For this review, take the finished solid that the model builds, in its own axes (mm). Face numbers are marked on the shaded views. A direction names the side the tool comes from. Round coordinates to 2 decimals unless told otherwise and drop trailing zeros. Order: outer loops, then holes, each group sorted by start corner. A loop starts at its lowest first (then second) coordinate and runs counter-clockwise, first axis right, second up. Notation, with made-up numbers: M 44.5,17 L 66.5,17 A31 ccw 66.5,43 Z; hole C 15.25,33.5 d6. An arc over 180 degrees is marked long. Use a Markdown table: item, result.
from build123d import *

# Parameters (mm, degrees)
F3_DEPTH = 25
F2_W     = 14.679278
F2_H     = 9.152961
F4_DEPTH = 25
F5_DEPTH = 25


with BuildPart() as f3:
    # F1 (on Front) → F3 (new body, symmetric)
    with BuildSketch(Plane.XZ):
        with BuildLine():
            Line((15.849059, 25), (-19.900017, 25))
            ThreePointArc((-19.900017, 25), (-23.663126, 21.043852), (-25, 15.75))
            Line((-25, 15.75), (-25, -13.906561))
            Line((-25, -13.906561), (-25, -14.566518))
            ThreePointArc((-25, -14.566518), (-21.671652, -22.024724), (-14.065702, -25))
            Line((-14.065702, -25), (15.273589, -25))
            ThreePointArc((15.273589, -25), (20.913091, -23.706775), (25, -19.611218))
            Line((25, -19.611218), (25, -9.521818))
            Line((25, -9.521818), (25, 15.948113))
            ThreePointArc((25, 15.948113), (22.284826, 22.35471), (15.849059, 25))
        make_face()
        with BuildLine():
            Line((-10.707237, -10.016448), (-10.707237, 0))
            Line((-10.707237, 0), (-10.707237, 10.016448))
            ThreePointArc((-10.707237, 10.016448), (-10.10992, 12.373308), (-8.462171, 14.161184))
            Line((-8.462171, 14.161184), (4.317435, 14.161184))
            Line((4.317435, 14.161184), (5.699014, 14.161184))
            ThreePointArc((5.699014, 14.161184), (8.629785, 12.947219), (9.843749, 10.016448))
            Line((9.843749, 10.016448), (9.843749, 0))
            Line((9.843749, 0), (9.843749, -10.016448))
            ThreePointArc((9.843749, -10.016448), (8.630455, -12.592476), (5.871711, -13.297698))
            Line((5.871711, -13.297698), (-6.907895, -13.297698))
            ThreePointArc((-6.907895, -13.297698), (-9.558442, -12.526508), (-10.707237, -10.016448))
        make_face(mode=Mode.SUBTRACT)
    extrude(amount=F3_DEPTH, both=True)

    # F2 (on Right) → F4 (intersect, symmetric)
    with BuildSketch(Plane.YZ):
        with BuildLine():
            Line((-25, -25), (-7.54655, -25))
            Line((-7.54655, -25), (-7.54655, -10.016448))
            Line((-7.54655, -10.016448), (6.960031, -10.016448))
            Line((6.960031, -10.016448), (6.960031, -25))
            Line((6.960031, -25), (25, -25))
            Line((25, -25), (25, 15.715461))
            ThreePointArc((25, 15.715461), (21.733554, 22.047274), (15.249502, 25))
            Line((15.249502, 25), (-15.145234, 25))
            ThreePointArc((-15.145234, 25), (-21.510489, 22.233155), (-25, 16.233554))
            Line((-25, 16.233554), (-25, -25))
        make_face()
        with Locations((-0.725002, 10.793585)):
            Rectangle(F2_W, F2_H, mode=Mode.SUBTRACT)
    extrude(amount=F4_DEPTH, both=True, mode=Mode.INTERSECT)

    # F0 (on Top) → F5 (intersect, symmetric)
    with BuildSketch(Plane.XY):
        Polygon((25, 25), (-25, 25), (-25, 16.938681), (-13, 16.938681), (-13, -17.136794), (-25, -17.136794), (-25, -25), (25, -25), (25, -16.344341), (13, -16.344341), (13, 16.542453), (25, 16.542453), align=None)
    extrude(amount=F5_DEPTH, both=True, mode=Mode.INTERSECT)


solid = f3.part
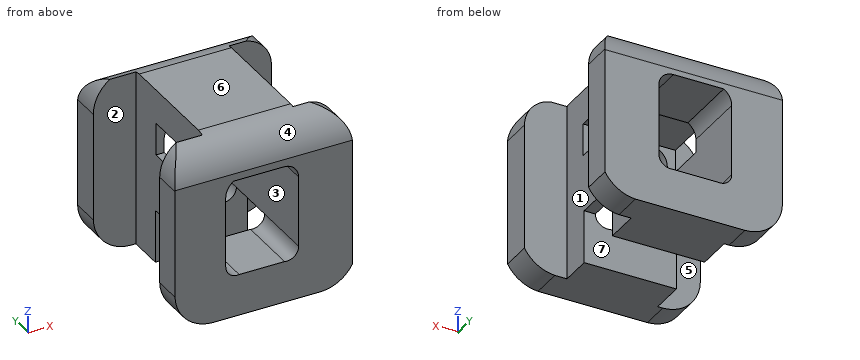
Q1. Draft analysis for pull direction Y (two halves, no side actions). For the marked faces 4, 5, 6 and 7, state which applies: pulls with the +Y half, pulls with the -Y half, needs draft (parallel to the pull), parting line crosses it, or undercut.
Determined:
| item | result |
|---|---|
| face 4 | pulls with the -Y half |
| face 5 | undercut |
| face 6 | needs draft |
| face 7 | undercut |
Q2. Wall thickness on line 1 along X through (y, z) = (9.5, -3); line 2 along Y through (x, z) = (16, 14.5); line 3 along Y through (x, z) = (-21, -2.5): over which ranges is each line inside the solid? List them lowest first. Write a range as [from, to].
Determined:
| item | result |
|---|---|
| line 1 | x = [-13, -10.71], [9.84, 13] |
| line 2 | y = [-25, -16.34], [16.54, 25] |
| line 3 | y = [-25, -17.14], [16.94, 25] |
Q3. Clearance check with flat-ended pins moving along their axes: pin 1 (16.5 mm diameter, centred on y = -0.5, z = -2.5, fed in from +X); pin 2 (4 mm diameter, centred on y = -5, z = 9.5, fed in from -X); pin 3 (2.5 mm diameter, centred on x = -12, y = 2.5, fed in from -Z); pin 4 (12 mm diameter, centred on x = 16, y = -17, fed in from +Z). State where each tip first meets the part, or that it passes through.
Determined:
| item | result |
|---|---|
| pin 1 | stops at x = 13 |
| pin 2 | passes through |
| pin 3 | stops at z = -10.02 |
| pin 4 | stops at z = 25 |
Q4. Machinability: for the marked faces 1, 2 and 3, which of the approach directions +Z, -Z, +X, -X, +Y, -Y give a long, thin tool a straight path to every point of the face, cutting with its end or side? Answer none if there is none.
Determined:
| item | result |
|---|---|
| face 1 | +Z, -Z, +X |
| face 2 | +Z, -Z, -X |
| face 3 | +Y, -Y |
Q5. Add section C-C (z = 5). Write out the cut boundary in (x, y), then the cut area to 3 significant figures.
Determined:
| item | result |
|---|---|
| outline | M -25,-25 L -10.71,-25 L -10.71,25 L -25,25 L -25,16.94 L -13,16.94 L -13,-17.14 L -25,-17.14 Z; M 9.84,-25 L 25,-25 L 25,-16.34 L 13,-16.34 L 13,16.54 L 25,16.54 L 25,25 L 9.84,25 Z |
| area | 669 mm^2 |
Q6. Add section A-A (x = -2.5). Write out the cut boundary in (y, z), then the cut area to 3 significant figures.
Determined:
| item | result |
|---|---|
| outline | M -25,-25 L -7.55,-25 L -7.55,-13.3 L -25,-13.3 Z; M -25,14.16 L -8.06,14.16 L -8.06,15.37 L 6.61,15.37 L 6.61,14.16 L 25,14.16 L 25,15.72 A10.88 ccw 15.25,25 L -15.15,25 A11.13 ccw -25,16.23 Z; M 6.96,-25 L 25,-25 L 25,-13.3 L 6.96,-13.3 Z |
| area | 892 mm^2 |
Q7. Add section B-B (y = 5.5). Write out the cut boundary in (x, z), then the cut area to 3 significant figures.
Determined:
| item | result |
|---|---|
| outline | M -13,-10.02 L -10.71,-10.02 L -10.71,6.22 L -13,6.22 Z; M -13,15.37 L 13,15.37 L 13,25 L -13,25 Z; M 9.84,-10.02 L 13,-10.02 L 13,6.22 L 9.84,6.22 Z |
| area | 339 mm^2 |
Q8. Add section D-D (x = -16). Write out the cut boundary in (y, z).
Determined:
| item | result |
|---|---|
| outline | M -25,-24.86 L -17.14,-24.86 L -17.14,24.63 A11.13 ccw -25,16.23 Z; M 16.94,-24.86 L 25,-24.86 L 25,15.72 A10.88 ccw 16.94,24.71 Z |
